Input: part model. Units: mm. Frame: model coordinates. A direction names the side the tool comes from. Round coordinates to 2 decimals unless told otherwise and drop trailing zeros. Loops run counter-clockwise (first coordinate to the right, second up) from the corner with the lowest first, then second, coordinate; pieces in that order, holes last.
1) Access query for faces 4 (the face through (-2.885, -8.425, -12.754)), 5 (the face through (-38.467, -13.911, -10.521)), 6 (the face through (-16, -22.01, -7)), 7 (the face through (-29, -2, -12.5)). Directions: +Z, -Z, +X, -X, +Y, -Y. A direction counts if a zero-diameter tool reaches every point of the face in a straight line with its end or side. Return the directions, or none.
2) First-contact query: pin 1 (0.6 mm diameter, centred on x = -3, z = -12.5, fed in from -Y); pin 2 (8.5 mm diameter, centred on x = -19.5, y = -35, fed in from +Z); pin 3 (5.5 mm diameter, centred on x = -0.5, y = -7, fed in from -Z); pin 4 (0.8 mm diameter, centred on y = -46.5, z = -12.5, fed in from +X). Flat tips, straight axial feed; report the tip coordinate or a pass-through.
3) Ray query, line 1 along Z through (x, y) = (-9, -16); line 2 along Z through (x, y) = (-40, 0); line 3 along Y through (x, z) = (-18, -8.5). Return the intervals inside material, ascending.
4) Section D-D, the plane z = -11. Return loops of the section in (x, y), and give its area (3 significant figures).
5) Draft query along X for faces 1 (the face through (-29.721, -2.916, -12.754)), 2 (the face through (-20.5, -24, -7)), 3 (the face through (-40, -1, -9)). Return one class per face: pulls with the +X half, pulls with the -X half, needs draft (parallel to the pull), parting line crosses it, or undercut.
6) Section C-C, the plane y = -44. Return loops of the section in (x, z), and give its area (3 significant figures).
7) Section A-A, the plane z = -4. Return loops of the section in (x, y).
8) Section B-B, the plane x = -39.85. Return loops of the section in (y, z).
from build123d import *

# Parameters (mm, degrees)
PAD037_DEPTH    = 1
SKETCH062_W     = 8.1
SKETCH062_H     = 3.05
SKETCH062_W_2   = 3.05
SKETCH062_H_2   = 8.1
POCKET025_DEPTH = 0.5
POCKET026_DEPTH = 0.25
POCKET027_DEPTH = 0.25
CHAMFER010_SIZE = 0.25
SKETCH065_W     = 9
SKETCH065_H     = 4
PAD038_DEPTH    = 12
SKETCH066_R     = 1.97
POCKET028_DEPTH = 29.6647358036
SKETCH067_R     = 1.45
PAD039_DEPTH    = 3
CHAMFER011_SIZE = 1


with BuildPart() as part:
    # Sketch061 (on Face2 of Binder016) → Pad037 (new body)
    with BuildSketch(Plane(origin=(0, 0, -13), x_dir=(1, 0, 0), z_dir=(0, 0, -1))):
        Polygon((-61, -3.6537388036), (-61, 44.999997), (-50.28, 44.999997), (-50.28, 47.899997), (-35.38, 47.899997), (-35.38, 44.999997), (-23.28025859, 44.999997), (-23.28025859, 47.899997), (-8.38025859, 47.899997), (-8.38025859, 44.999997), (-2.14025859, 44.999997), (-2.14025859, 9.80692559), (3.5165956595, 4.1500713405), (-21.4834043405, 4.1500713405), (-35, -3.6537388036), align=None)
    extrude(amount=-PAD037_DEPTH)

    # Sketch062 (on Face16 of Pad037) → Pocket025 (cut)
    with BuildSketch(Plane(origin=(0, 0, -13), x_dir=(1, 0, 0), z_dir=(0, 0, -1))):
        with Locations((-51, -2.1287388036)):
            Rectangle(SKETCH062_W, SKETCH062_H)
        with Locations((-8.9834043405, 5.6750713405)):
            Rectangle(SKETCH062_W, SKETCH062_H)
        with Locations((-3.66525859, 16.80692559)):
            Rectangle(SKETCH062_W_2, SKETCH062_H_2)
        with Locations((-3.66525859, 37.999997)):
            Rectangle(SKETCH062_W_2, SKETCH062_H_2)
        Polygon((1.0770772644, 6.5895897356), (-1.8220605384, 9.4887275384), (-3.9787362211, 7.3320518558), (-1.0795984182, 4.432914053), align=None)
        Polygon((-31.752404736, -1.7787388033), (-24.7375989657, 2.2712611973), (-26.2625989659, 4.9126386787), (-33.2774047362, 0.8626386781), align=None)
    extrude(amount=-POCKET025_DEPTH, mode=Mode.SUBTRACT)

    # Sketch063 (on Face5 of Pocket025) → Pocket026 (cut)
    with BuildSketch(Plane.XY.offset(-12)):
        Polygon((-2.14025859, -44.999997), (-2.14025859, -9.80692559), (3.5165956595, -4.1500713405), (2.8094888783, -4.1500713405), (-2.64025859, -9.5998188088), (-2.64025859, -44.999997), align=None)
    extrude(amount=-POCKET026_DEPTH, mode=Mode.SUBTRACT)

    # Sketch064 (on Face5 of Pocket026) → Pocket027 (cut)
    with BuildSketch(Plane.XY.offset(-12)):
        Polygon((-2.64025859, -29.449997), (-42.5062839938, -29.449997), (-61, -18.7726450855), (-61, -19.3499953547), (-42.64025859, -29.949997), (-2.64025859, -29.949997), align=None)
    extrude(amount=-POCKET027_DEPTH, mode=Mode.SUBTRACT)

    # Chamfer010
    chamfer010_edges = [part.edges().sort_by_distance(p)[0] for p in [
        (-61, -32.174996, -12),
        (-61, -7.559453, -12),
    ]]
    chamfer(chamfer010_edges, length=CHAMFER010_SIZE)

    # Sketch065 (on Face46 of Chamfer010) → Pad038 (join)
    with BuildSketch(Plane.XY.offset(-12)):
        with Locations((-16.00025859, -24.009997)):
            Rectangle(SKETCH065_W, SKETCH065_H)
    extrude(amount=PAD038_DEPTH)

    # Sketch066 (on Face54 of Pad038) → Pocket028 (cut, through all)
    with BuildSketch(Plane.XZ.offset(26.009997)):
        with Locations((-16.00025859, -4)):
            Circle(SKETCH066_R)
    extrude(amount=-POCKET028_DEPTH, mode=Mode.SUBTRACT)

    # Sketch067 (on Face46 of Pocket028) → Pad039 (join)
    with BuildSketch(Plane.XY.offset(-12)):
        with Locations((-39.85, -1.3462611964)):
            Circle(SKETCH067_R)
        with Locations((-39.85, -14.3462611964)):
            Circle(SKETCH067_R)
    extrude(amount=PAD039_DEPTH)

    # Chamfer011
    chamfer011_edges = [part.edges().sort_by_distance(p)[0] for p in [
        (-11.500259, -26.009997, -6),
        (-16.000259, -26.009997, 0),
        (-20.500259, -26.009997, -6),
        (-20.500259, -24.009997, 0),
        (-16.000259, -22.009997, 0),
        (-11.500259, -24.009997, 0),
        (-11.500259, -22.009997, -6),
        (-20.500259, -22.009997, -6),
    ]]
    chamfer(chamfer011_edges, length=CHAMFER011_SIZE)


solid = part.part
Final values:
1. face 4: -Z, +X
1. face 5: +Z
1. face 6: +Z, +X, -X, +Y
1. face 7: -Z
2. pin 1: stops at y = -45
2. pin 2: stops at z = -12
2. pin 3: stops at z = -13
2. pin 4: stops at x = -8.38
3. line 1: z = -13 to -12
3. line 2: z = -13 to -9
3. line 3: y = -26.01 to -22.01
4. outline: circle Ø2.9 at (-39.85, -14.35); circle Ø2.9 at (-39.85, -1.35); (-20.5, -25.01) - (-19.5, -26.01) - (-12.5, -26.01) - (-11.5, -25.01) - (-11.5, -23.01) - (-12.5, -22.01) - (-19.5, -22.01) - (-20.5, -23.01) - close
4. area: 47.2 mm2
5. face 1: undercut
5. face 2: pulls with the -X half
5. face 3: needs draft
6. outline: (-61, -13) - (-2.14, -13) - (-2.14, -12.25) - (-2.64, -12.25) - (-2.64, -12) - (-60.75, -12) - (-61, -12.25) - close
6. area: 58.7 mm2
7. outline: (-20.5, -25.01) - (-19.5, -26.01) - (-17.97, -26.01) - (-17.97, -22.01) - (-19.5, -22.01) - (-20.5, -23.01) - close; (-14.03, -26.01) - (-12.5, -26.01) - (-11.5, -25.01) - (-11.5, -23.01) - (-12.5, -22.01) - (-14.03, -22.01) - close
8. outline: (-47.9, -13) - (3.65, -13) - (3.65, -12) - (0.1, -12) - (0.1, -9) - (-2.8, -9) - (-2.8, -12) - (-12.9, -12) - (-12.9, -9) - (-15.8, -9) - (-15.8, -12) - (-29.45, -12) - (-29.45, -12.25) - (-29.95, -12.25) - (-29.95, -12) - (-47.9, -12) - close
